from build123d import *

# Parameters (mm, degrees)
F0_W     = 711.2
F0_H     = 38.1
F1_DEPTH = 19.05
F3_D     = 11.50874
F5_D     = 25.4508
F6_W     = 6.5565072059
F6_H     = 2.54
F7_DEPTH = 19.051
F9_D     = 12.7


with BuildPart() as f1:
    # F0 (on Top) → F1 (new body)
    with BuildSketch(Plane.XY):
        with Locations((-168.5031287369, 0)):
            Rectangle(F0_W, F0_H)
    extrude(amount=F1_DEPTH)

    # F3 (through all)
    with Locations(Plane.XY.offset(19.05)):
        with Locations((-143.1031287369, 0), (-117.7031287369, 0), (-92.3031287369, 0), (-66.9031287369, 0), (-16.1031287369, 0), (-41.5031287369, 0), (9.2968712631, 0), (34.6968712631, 0), (60.0968712631, 0), (85.4968712631, 0), (-168.5031287369, 0), (-193.9031287369, 0), (110.8968712631, 0), (136.2968712631, 0), (161.6968712631, 0)):
            Hole(F3_D / 2)

    # F5 (through all)
    with Locations(Plane.XY.offset(19.05)):
        with Locations((-492.3531287369, 0)):
            Hole(F5_D / 2)

    # F6 (on face) → F7 (cut, through all)
    with BuildSketch(Plane.XY.offset(19.05)):
        with Locations((-527.3813823399, 0)):
            Rectangle(F6_W, F6_H)
        with BuildLine():
            Line((-494.1921649058, 1.27), (-505.0149968913, 1.27))
            ThreePointArc((-505.0149968913, 1.27), (-505.0785287369, 0), (-505.0149968913, -1.27))
            Line((-505.0149968913, -1.27), (-494.1921649058, -1.27))
            Line((-494.1921649058, -1.27), (-494.1921649058, 1.27))
        make_face()
        with BuildLine():
            Line((-505.0149968913, 1.27), (-524.1031287369, 1.27))
            Line((-524.1031287369, 1.27), (-524.1031287369, -1.27))
            Line((-524.1031287369, -1.27), (-505.0149968913, -1.27))
            ThreePointArc((-505.0149968913, -1.27), (-505.0785287369, 0), (-505.0149968913, 1.27))
        make_face()
    extrude(amount=-F7_DEPTH, mode=Mode.SUBTRACT)

    # F9 (through all)
    with Locations(Plane(origin=(0, 19.05, 0), x_dir=(-1, 0, 0), z_dir=(0, 1, 0))):
        with Locations((513.9431287369, 9.525)):
            Hole(F9_D / 2)


solid = f1.part
Check sheet for the modelled part. Datum: model origin and axes. Units: mm. A direction names the side the tool comes from. Round coordinates to 2 decimals unless told otherwise and drop trailing zeros. One line per item, written item: value.
(1) Access from +Z, -Z, +X, -X, +Y, -Y to the whole of each face (thin tool, end or side, straight path). Record for faces 1 (the face through (-519, 1.27, 14)), 2 (the face through (105.4, 1.7, 9.4)).
Computed values:
face 1: +Z, -Z, -X
face 2: +Z, -Z
(2) Thickness scan on line 1 (Y direction, x = -41.5, z = 14.5); line 2 (X direction, y = 11, z = 14); line 3 (X direction, y = -16, z = 10.5). Record the ranges inside material, lowest first.
Computed values:
line 1: y = -19.05 to -5.75, 5.75 to 19.05
line 2: x = -524.1 to -518.45, -509.44 to -498.75, -485.96 to 187.1
line 3: x = -524.1 to -520.22, -507.67 to 187.1
(3) Release check for a two-part mould opening along X. For faces 3 (the face through (65.846, 0.253, 9.392)), 4 (the face through (-524.103, -10, 9)), 5 (the face through (-173, 19.05, 9)) record: +X half, -X half, draft (parallel to the pull), parting line (faces both ways), or undercut.
Computed values:
face 3: undercut
face 4: -X half
face 5: draft
